Could you check a few things on this drawing? It's one solid part, dimensions in mm from its lowest x, y, z. A direction names the side the tool comes from. Give positions to 0.01 mm unless a question says otherwise; leave off trailing zeros. Loops run counter-clockwise (first coordinate to the right, second up) from the corner with the lowest first, then second, coordinate; pieces in that order, holes last. Notation, with made-up numbers: M 27.25,86.25 L 75.25,86.25 A21 cw 75.25,90.25 Z; hole C 6.25,-24 d3. An arc over 180 degrees is marked long. Return JSON: item names as keys, results as strings. Group by question number.
1. For pin 1 (4 mm diameter, centred on y = 12.5, z = 21.5, fed in from +X); pin 2 (8 mm diameter, centred on x = 22, y = 11, fed in from -Z) (1 decimal), each with a flat end and sliding along its axis, tell me the tip position at first contact or that it passes through.
2. For the marked faces 1 and 2, which set-ups out of +Z, -Z, +X, -X, +Y, -Y let a thin tool reach every point of the face, with its end or its side?
3. If we section it at B-B (z = 12.7): Write out the boundary of the cut face in (x, y).
4. If we section it at D-D (y = 43.5): Write out the boundary of the cut face in (x, z) (1 decimal).
5. If we section it at C-C (y = 20.5): Write out the boundary of the cut face in (x, z) (1 decimal).
6. Please list where these lines run through material, in increasing order: line 1 (Y direction, x = 57.15, z = 7); line 2 (X direction, y = 16.5, z = 1.75) (1 decimal); line 3 (Y direction, x = 54, z = 3).
7. If we mould it in two halves opening along X, with no side actions, what happens to the marked faces 3, 4, 5 and 6? For each: +X half, -X half, draft (parallel to the pull), parting line (faces both ways), or undercut.
8. If we section it at A-A (x = 57.15): Write out the boundary of the cut face in (y, z).
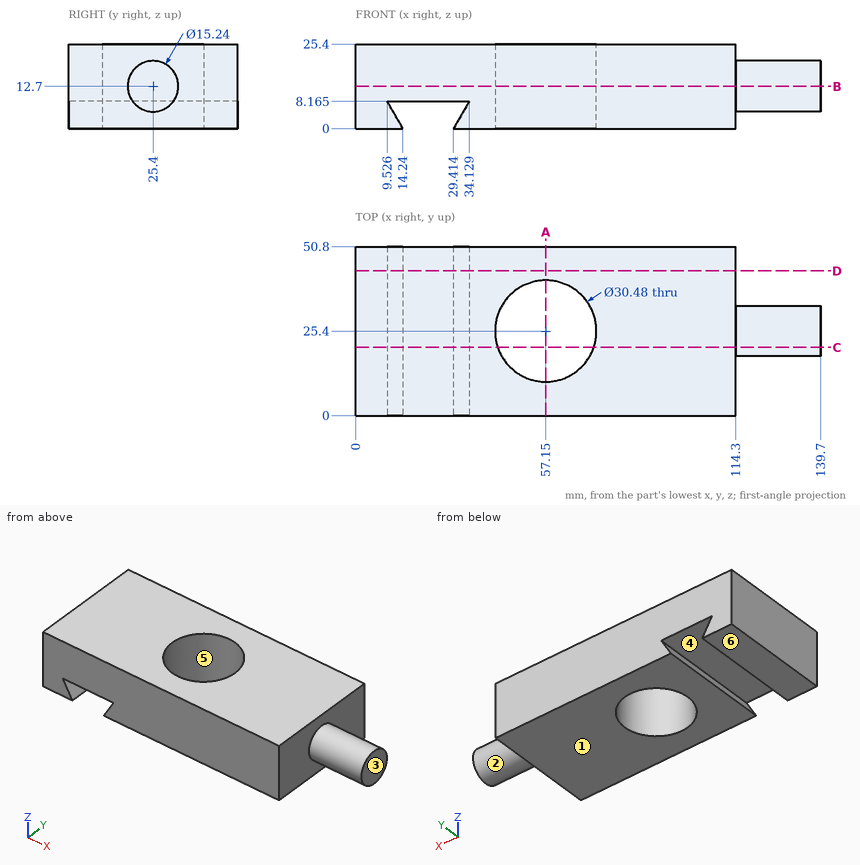
Answer:
{
 "1": {"pin 1": "stops at x = 114.3", "pin 2": "stops at z = 8.2"},
 "2": {"face 1": "-Z, +X, -X, +Y, -Y", "face 2": "+X"},
 "3": {"outline": "M 0,0 L 114.3,0 L 114.3,17.78 L 139.7,17.78 L 139.7,33.02 L 114.3,33.02 L 114.3,50.8 L 0,50.8 Z; hole C 57.15,25.4 d30.48"},
 "4": {"outline": "M 0,0 L 14.2,0 L 9.5,8.2 L 34.1,8.2 L 29.4,0 L 114.3,0 L 114.3,25.4 L 0,25.4 Z"},
 "5": {"outline": "M 0,0 L 14.2,0 L 9.5,8.2 L 34.1,8.2 L 29.4,0 L 42.7,0 L 42.7,25.4 L 0,25.4 Z; M 71.6,0 L 114.3,0 L 114.3,6.9 L 139.7,6.9 L 139.7,18.5 L 114.3,18.5 L 114.3,25.4 L 71.6,25.4 Z"},
 "6": {"line 1": "y = 0 to 10.16, 40.64 to 50.8", "line 2": "x = 0 to 13.2, 30.4 to 44.8, 69.5 to 114.3", "line 3": "y = 0 to 10.49, 40.31 to 50.8"},
 "7": {"face 3": "+X half", "face 4": "undercut", "face 5": "undercut", "face 6": "draft"},
 "8": {"outline": "M 0,0 L 10.16,0 L 10.16,25.4 L 0,25.4 Z; M 40.64,0 L 50.8,0 L 50.8,25.4 L 40.64,25.4 Z"}
}
